```python
from build123d import *

# Parameters (mm, degrees)
SKETCH1_W           = 98
SKETCH1_H           = 21.59
BOSS_EXTRUDE1_DEPTH = 4
SKETCH2_W           = 98
SKETCH2_H           = 4
BOSS_EXTRUDE2_DEPTH = 40
SKETCH3_R           = 0.8
CUT_EXTRUDE1_DEPTH  = 21
FILLET1_R           = 1
SKETCH4_R           = 1
CUT_EXTRUDE2_DEPTH  = 21


with BuildPart() as part:
    # Sketch1 → Boss-Extrude1 (new body)
    with BuildSketch(Plane(origin=(0, 0, 0), x_dir=(1, 0, 0), z_dir=(0, 1, 0))):
        Rectangle(SKETCH1_W, SKETCH1_H)
    extrude(amount=BOSS_EXTRUDE1_DEPTH)

    # Sketch2 → Boss-Extrude2 (add)
    with BuildSketch(Plane(origin=(0, 4, 0), x_dir=(1, 0, 0), z_dir=(0, 1, 0))):
        with Locations((0, 8.795)):
            Rectangle(SKETCH2_W, SKETCH2_H)
    extrude(amount=BOSS_EXTRUDE2_DEPTH)

    # Sketch3 → Cut-Extrude1 (cut)
    with BuildSketch(Plane.XY.offset(-6.795)):
        with Locations((-39.5, 6.904051391)):
            Circle(SKETCH3_R)
        with Locations((-39.5, 36.904051391)):
            Circle(SKETCH3_R)
        with Locations((39.5, 36.904051391)):
            Circle(SKETCH3_R)
        with Locations((39.5, 6.904051391)):
            Circle(SKETCH3_R)
    extrude(amount=-CUT_EXTRUDE1_DEPTH, mode=Mode.SUBTRACT)

    # Fillet1
    fillet1_edges = [part.edges().sort_by_distance(p)[0] for p in [
        (0, 4, -6.795),
        (49, 44, -8.795),
        (-49, 44, -8.795),
        (0, 0, -10.795),
        (49, 2, 10.795),
        (-49, 2, 10.795),
    ]]
    fillet(fillet1_edges, radius=FILLET1_R)

    # Sketch4 → Cut-Extrude2 (cut)
    with BuildSketch(Plane(origin=(0, 4, 0), x_dir=(1, 0, 0), z_dir=(0, 1, 0))):
        with Locations((-34, -2)):
            Circle(SKETCH4_R)
        with Locations((34, -2)):
            Circle(SKETCH4_R)
    extrude(amount=-CUT_EXTRUDE2_DEPTH, mode=Mode.SUBTRACT)


solid = part.part
```
For this review, take the finished solid that the model builds, in its own axes (mm). A direction names the side the tool comes from. Coordinates: 2 decimals unless noted, no trailing zeros. Write each loop counter-clockwise with the first axis right and the second up, starting at its lowest first coordinate (ties: lowest second). Pieces come first, ordered by that corner, then holes.
(1) Tool access review of faces 5 (the face through (-1, 44, -9)), 6 (the face through (-1, 4, 2)): name each direction out of +Z, -Z, +X, -X, +Y, -Y from which nothing blocks a thin tool from reaching the whole face with its end or side.
(2) Add section A-A on x = -34. Give the boundary of the cut face in (y, z) (3 decimals).
(3) Add section D-D on y = 22. Give the boundary of the cut face in (x, z) (3 decimals), then the cut area to 3 significant figures.
(4) Add section C-C on x = 41.5. Give the boundary of the cut face in (y, z) (3 decimals), then the cut area to 3 significant figures.
(5) For pin 1 Ø2.5 at (x, y) = (39.5, 6.9) entering from +Z (3 decimals), flat-tipped, find the tip position at first contact; note if it passes through.
(6) The part is to be moulded in two halves that separate along Z. For faces 1 (the face through (-1, 22, -10.795)), 2 (the face through (-1, 24, -6.795)), 3 (the face through (-49, 15, -7)), 4 (the face through (33.263, 2.028, 1.324)), say which applies: +Z half, -Z half, draft (parallel to the pull), parting line (faces both ways), or undercut.
(7) Add section B-B on z = 2. Give the boundary of the cut face in (x, y), then the cut area to 3 significant figures.
(8) Wall thickness on probe 1 along X at (y, z) = (2.8, 2); probe 2 along Y at (x, z) = (-39.5, -9.8); probe 3 along Z at (x, y) = (34, 1.6) (3 decimals): over which ranges is each line inside the solid? List them lowest first.
Answer sheet:
1. face 5: +Z, -Z, +X, -X, +Y
1. face 6: +Z, +X, -X, +Y
2. outline: (0, -9.795) arc R1 ccw to (1, -10.795) - (44, -10.795) - (44, -6.795) - (5, -6.795) arc R1 cw to (4, -5.795) - (4, 1) - (0, 1) - close; (0, 3) - (4, 3) - (4, 10.795) - (0, 10.795) - close
3. outline: (-49, -10.795) - (49, -10.795) - (49, -6.795) - (-49, -6.795) - close
3. area: 392 mm2
4. outline: (0, -9.795) arc R1 ccw to (1, -10.795) - (44, -10.795) - (44, -6.795) - (5, -6.795) arc R1 cw to (4, -5.795) - (4, 10.795) - (0, 10.795) - close
4. area: 246 mm2
5. pin 1: stops at z = -6.795
6. face 1: -Z half
6. face 2: +Z half
6. face 3: draft
6. face 4: undercut
7. outline: (-49, 0) - (-35, 0) - (-35, 4) - (-49, 4) - close; (-33, 0) - (33, 0) - (33, 4) - (-33, 4) - close; (35, 0) - (49, 0) - (49, 4) - (35, 4) - close
7. area: 376 mm2
8. probe 1: x = -49 to -35, -33 to 33, 35 to 49
8. probe 2: y = 0 to 6.1, 7.7 to 36.1, 37.7 to 44
8. probe 3: z = -10.795 to 1, 3 to 10.795
